```python
from build123d import *

# Parameters (mm, degrees)
BOSS_EXTRUDE1_DEPTH = 15
FILLET1_R           = 10
FILLET3_R           = 2
FILLET6_R           = 2.5


with BuildPart() as part:
    # Sketch1 → Boss-Extrude1 (new body)
    with BuildSketch(Plane(origin=(0, 0, 0), x_dir=(1, 0, 0), z_dir=(0, 1, 0))):
        with BuildLine():
            Line((65, -75), (80.311288741, -75))
            ThreePointArc((80.311288741, -75), (42.504840348, -115.233391292), (0, -80))
            Line((0, -80), (0, -50))
            Line((0, -50), (0, 0))
            Line((0, 0), (0, 15))
            Line((0, 15), (80, 15))
            Line((80, 15), (80, 0))
            Line((80, 0), (80, -20))
            Line((80, -20), (65, -20))
            Line((65, -20), (65, -18.5))
            ThreePointArc((65, -18.5), (64, -17.5), (65, -16.5))
            Line((65, -16.5), (65, -13.5))
            ThreePointArc((65, -13.5), (64, -12.5), (65, -11.5))
            Line((65, -11.5), (65, -8.5))
            ThreePointArc((65, -8.5), (64, -7.5), (65, -6.5))
            Line((65, -6.5), (65, -3.5))
            ThreePointArc((65, -3.5), (64, -2.5), (65, -1.5))
            Line((65, -1.5), (65, 0))
            Line((65, 0), (15, 0))
            Line((15, 0), (15, -50))
            Line((15, -50), (15, -75))
            ThreePointArc((15, -75), (40, -100), (65, -75))
        make_face()
    extrude(amount=BOSS_EXTRUDE1_DEPTH)

    # Fillet1
    fillet1_edges = [part.edges().sort_by_distance(p)[0] for p in [
        (0, 7.5, -15),
        (80, 7.5, -15),
    ]]
    fillet(fillet1_edges, radius=FILLET1_R)

    # Fillet3
    # the kernel refuses this fillet: 2 mm, written as the material it takes off along each edge
    with BuildSketch(Plane(origin=(80, -5, 20), x_dir=(0, 0, -1), z_dir=(0, 1, 0))) as fillet3_piece_1:
        with BuildLine():
            CenterArc((FILLET3_R, FILLET3_R), FILLET3_R, 180, 90)
            Line((0, FILLET3_R), (-FILLET3_R * 0.02, FILLET3_R))
            Line((-FILLET3_R * 0.02, FILLET3_R), (-FILLET3_R * 0.02, -FILLET3_R * 0.02))
            Line((-FILLET3_R * 0.02, -FILLET3_R * 0.02), (FILLET3_R, -FILLET3_R * 0.02))
            Line((FILLET3_R, -FILLET3_R * 0.02), (FILLET3_R, 0))
        make_face()
    extrude(amount=25, mode=Mode.SUBTRACT)
    with BuildSketch(Plane(origin=(65, -4.841229183, 20), x_dir=(1, 0, 0), z_dir=(0, 1, 0))) as fillet3_piece_2:
        with BuildLine():
            CenterArc((1.936491673, 2), FILLET3_R, 194.477512186, 75.522487814)
            Line((0, 1.5), (-0.038729833, 1.49))
            ThreePointArc((-0.038729833, 1.49), (-0.04, 0.75), (-0.04, 0))
            Line((-0.04, 0), (0, -0.04))
            Line((0, -0.04), (1.936491673, -0.04))
            Line((1.936491673, -0.04), (1.936491673, 0))
        make_face()
    extrude(amount=24.682458366, mode=Mode.SUBTRACT)

    # Fillet6
    fillet6_edges = [part.edges().sort_by_distance(p)[0] for p in [
        (65, 7.5, 75),
        (80.311288741, 7.5, 75),
    ]]
    fillet(fillet6_edges, radius=FILLET6_R)


solid = part.part
```
The model under review builds one solid part; all positions refer to its coordinate system, in mm. A direction names the side the tool comes from. Coordinates: 2 decimals unless noted, no trailing zeros. Write each loop counter-clockwise with the first axis right and the second up, starting at its lowest first coordinate (ties: lowest second). Pieces come first, ordered by that corner, then holes.
1) The part is to be moulded in two halves that separate along Z. For faces 1 (the face through (40, 7, -15)), 2 (the face through (15, 7, 37)), 3 (the face through (42, 7.4, 115.26)), 4 (the face through (72, 7, 75)), say which applies: pulls with the +Z half, pulls with the -Z half, needs draft (parallel to the pull), parting line crosses it, or undercut.
2) We need section A-A on x = 40. State the section outline as (y, z) points.
3) Machinability: for faces 5 (the face through (80, 7, 6)), 6 (the face through (79.57, 7.6, 75.81)), 7 (the face through (40, 7, 0)), which of the approach directions +Z, -Z, +X, -X, +Y, -Y give a long, thin tool a straight path to every point of the face, cutting with its end or side? Answer none if there is none.
4) We need section C-C on z = 82.5. State the section outline as (x, y) points.
5) To check wall thickness, follow probe 1 along Z at (x, y) = (60, 12.5); probe 2 along Z at (x, y) = (23.5, 13); probe 3 along X at (y, z) = (1.75, 65). State the ranges of each line that lie inside material, in increasing order.
6) Clearance check with flat-ended pins moving along their axes: pin 1 Ø7.5 at (y, z) = (5.5, 6) entering from +X; pin 2 Ø9 at (x, y) = (73.5, 4) entering from +Z; pin 3 Ø1 at (x, y) = (18, 10.5) entering from +Z. State where each tip first meets the part, or that it passes through.
7) We need section D-D on z = 47. State the section outline as (x, y) points.
8) We need section B-B on y = 7.5. State the section outline as (x, z) points.
Answer list:
1. face 1: pulls with the -Z half
1. face 2: undercut
1. face 3: pulls with the +Z half
1. face 4: undercut
2. outline: (0, -15) - (15, -15) - (15, 0) - (0, 0) - close; (0, 100) - (15, 100) - (15, 115.31) - (0, 115.31) - close
3. face 5: -Z, +X, +Y, -Y
3. face 6: +X, +Y, -Y
3. face 7: +Y, -Y
4. outline: (0.39, 0) - (16.15, 0) - (16.15, 15) - (0.39, 15) - close; (63.85, 0) - (79.61, 0) - (79.61, 15) - (63.85, 15) - close
5. probe 1: z = -15 to 0, 90 to 110
5. probe 2: z = -15 to 0, 93.78 to 111.78
5. probe 3: x = 0 to 15
6. pin 1: stops at x = 80
6. pin 2: stops at z = 103
6. pin 3: stops at z = 109.1
7. outline: (0, 0) - (15, 0) - (15, 15) - (0, 15) - close
8. outline: (0, -5) arc R10 ccw to (10, -15) - (70, -15) arc R10 ccw to (80, -5) - (80, 18) arc R2 ccw to (78, 20) - (66.94, 20) arc R2 ccw to (65, 18.5) arc R1 ccw to (65, 16.5) - (65, 13.5) arc R1 ccw to (65, 11.5) - (65, 8.5) arc R1 ccw to (65, 6.5) - (65, 3.5) arc R1 ccw to (65, 1.5) - (65, 0) - (15, 0) - (15, 75) arc R25 cw to (64.9, 77.27) arc R2.5 ccw to (67.39, 75) - (77.73, 75) arc R2.5 ccw to (80.22, 77.67) arc R40.31 ccw to (0, 80) - close
